Read the model definition and answer for the solid it produces. Units are mm, in the model's axes. Give positions to 0.01 mm unless a question says otherwise; leave off trailing zeros. Write each loop counter-clockwise with the first axis right and the second up, starting at its lowest first coordinate (ties: lowest second). Pieces come first, ordered by that corner, then holes.
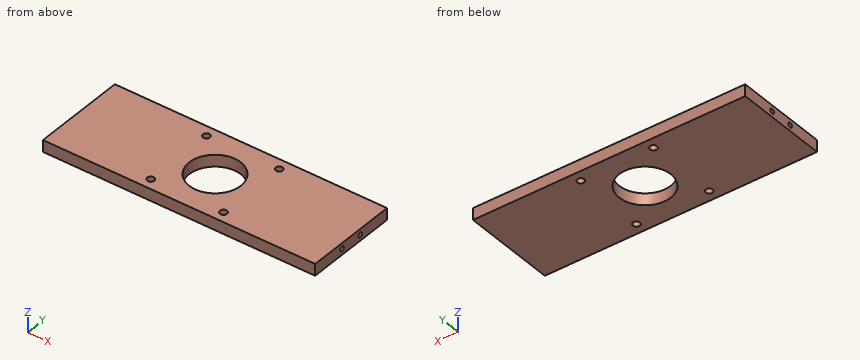
```python
from build123d import *

# Parameters (mm, degrees)
SKETCH1_W           = 116
SKETCH1_H           = 40
SKETCH1_R           = 11
SKETCH1_R_2         = 1.5
BOSS_EXTRUDE2_DEPTH = 5
SKETCH4_R           = 1
CUT_EXTRUDE1_DEPTH  = 10
SKETCH6_R           = 1
CUT_EXTRUDE2_DEPTH  = 5


with BuildPart() as part:
    # Sketch1 → Boss-Extrude2 (new body)
    with BuildSketch(Plane.XY):
        Rectangle(SKETCH1_W, SKETCH1_H)
        Circle(SKETCH1_R, mode=Mode.SUBTRACT)
        with Locations((-15.5, 15.5)):
            Circle(SKETCH1_R_2, mode=Mode.SUBTRACT)
        with Locations((-15.5, -15.5)):
            Circle(SKETCH1_R_2, mode=Mode.SUBTRACT)
        with Locations((15.5, -15.5)):
            Circle(SKETCH1_R_2, mode=Mode.SUBTRACT)
        with Locations((15.5, 15.5)):
            Circle(SKETCH1_R_2, mode=Mode.SUBTRACT)
    extrude(amount=BOSS_EXTRUDE2_DEPTH)

    # Sketch4 → Cut-Extrude1 (cut)
    with BuildSketch(Plane(origin=(58, 0, 0), x_dir=(0, 0, -1), z_dir=(1, 0, 0))):
        with Locations((-2.5, -5)):
            Circle(SKETCH4_R)
        with Locations((-2.5, 5)):
            Circle(SKETCH4_R)
    extrude(amount=-CUT_EXTRUDE1_DEPTH, mode=Mode.SUBTRACT)

    # Sketch6 → Cut-Extrude2 (cut)
    with BuildSketch(Plane.ZY.offset(58)):
        with Locations((2.5, 5)):
            Circle(SKETCH6_R)
        with Locations((2.5, -5)):
            Circle(SKETCH6_R)
    extrude(amount=-CUT_EXTRUDE2_DEPTH, mode=Mode.SUBTRACT)


solid = part.part
```
Item 1: Section A-A (x = 0) is taken. Write down the section's boundary in (y, z).
Result set:
outline: (-20, 0) - (-11, 0) - (-11, 5) - (-20, 5) - close; (11, 0) - (20, 0) - (20, 5) - (11, 5) - close
Item 2: Section C-C (z = 2.5) is taken. Write down the section's boundary in (x, y), and give its area (3 significant figures).
Result set:
outline: (-58, -20) - (58, -20) - (58, -6) - (48, -6) - (48, -4) - (58, -4) - (58, 4) - (48, 4) - (48, 6) - (58, 6) - (58, 20) - (-58, 20) - (-58, 6) - (-53, 6) - (-53, 4) - (-58, 4) - (-58, -4) - (-53, -4) - (-53, -6) - (-58, -6) - close; hole circle Ø3 at (-15.5, -15.5); hole circle Ø3 at (-15.5, 15.5); hole circle Ø22 at (0, 0); hole circle Ø3 at (15.5, -15.5); hole circle Ø3 at (15.5, 15.5)
area: 4,170 mm2
Item 3: Each of these flat-tipped pins is pushed along its axis until it touches: pin 1 Ø3.5 at (x, y) = (-15.5, -15.5) entering from -Z; pin 2 Ø1.6 at (y, z) = (5, 2.5) entering from +X; pin 3 Ø1.8 at (y, z) = (5, 2.5) entering from -X. Where does it stop, or does it pass through?
Result set:
pin 1: stops at z = 0
pin 2: stops at x = 48
pin 3: stops at x = -53
Item 4: Section D-D (x = -15.5) is taken. Write down the section's boundary in (y, z), and give its area (3 significant figures).
Result set:
outline: (-20, 0) - (-17, 0) - (-17, 5) - (-20, 5) - close; (-14, 0) - (14, 0) - (14, 5) - (-14, 5) - close; (17, 0) - (20, 0) - (20, 5) - (17, 5) - close
area: 170 mm2
Item 5: Section B-B (y = -15.5) is taken. Write down the section's boundary in (x, z).
Result set:
outline: (-58, 0) - (-17, 0) - (-17, 5) - (-58, 5) - close; (-14, 0) - (14, 0) - (14, 5) - (-14, 5) - close; (17, 0) - (58, 0) - (58, 5) - (17, 5) - close
Item 6: Find the intervals of material crossed by line 1 along Y through (x, z) = (-15.5, 2.95); line 2 along Y through (x, z) = (54, 2.5); line 3 along X through (y, z) = (2, 4.8), in increasing order.
Result set:
line 1: y = -20 to -17, -14 to 14, 17 to 20
line 2: y = -20 to -6, -4 to 4, 6 to 20
line 3: x = -58 to -10.82, 10.82 to 58
